Can you work these out from the model? Positions are in its coordinate system, mm. Round coordinates to 2 decimals unless told otherwise and drop trailing zeros. Order: outer loops, then holes, each group sorted by start corner. A loop starts at its lowest first (then second) coordinate and runs counter-clockwise, first axis right, second up. Notation, with made-up numbers: M -15,53 L 14,53 A11 ccw 14,74 Z; hole C 82.25,24.5 d3. An arc over 180 degrees is marked long. Answer as CSV lines item,"result". Start each with the question number.
from build123d import *

# Parameters (mm, degrees)
SKETCH1_W                   = 19.05
SKETCH1_H                   = 19.05
SKETCH1_W_2                 = 15.875
SKETCH1_H_2                 = 15.875
BOSS_EXTRUDE1_DEPTH         = 152.4
SKETCH2_R                   = 2.8956
BASEPLATE_MOUNT_HOLE_DEPTH  = 20.05
PS_BRACKET_MOUNT_HOLE_REACH = 21.05
SKETCH3_R                   = 4.7625
CUT_EXTRUDE1_REACH          = 21.05
SKETCH4_R                   = 4.7625
CUT_EXTRUDE2_REACH          = 21.05
SKETCH5_R                   = 4.7625


with BuildPart() as part:
    # Sketch1 → Boss-Extrude1 (new body, symmetric)
    with BuildSketch(Plane(origin=(0, 0, 0), x_dir=(0, -1, 0), z_dir=(0, 0, 1))):
        Rectangle(SKETCH1_W, SKETCH1_H)
        Rectangle(SKETCH1_W_2, SKETCH1_H_2, mode=Mode.SUBTRACT)
    extrude(amount=BOSS_EXTRUDE1_DEPTH, both=True)

    # Sketch2 → Baseplate Mount Hole (cut, through all)
    with BuildSketch(Plane(origin=(0, 9.525, 0), x_dir=(1, 0, 0), z_dir=(0, 1, 0))):
        with Locations((0, -114.3)):
            Circle(SKETCH2_R)
    extrude(amount=-BASEPLATE_MOUNT_HOLE_DEPTH, mode=Mode.SUBTRACT)

    # Sketch3 → PS Bracket Mount Hole (cut, up to next)
    with BuildSketch(Plane.ZY.offset(9.525), mode=Mode.PRIVATE) as ps_bracket_mount_hole_sk1:
        with Locations((-44.45, 0)):
            Circle(SKETCH3_R)
    ps_bracket_mount_hole_tool1 = extrude(ps_bracket_mount_hole_sk1.sketch, amount=-PS_BRACKET_MOUNT_HOLE_REACH, mode=Mode.PRIVATE) & part.part
    add(ps_bracket_mount_hole_tool1.solids().sort_by_distance((-9.525, 0, -44.45))[0], mode=Mode.SUBTRACT)

    # Sketch4 → Cut-Extrude1 (cut, up to next)
    with BuildSketch(Plane(origin=(0, 9.525, 0), x_dir=(1, 0, 0), z_dir=(0, 1, 0)), mode=Mode.PRIVATE) as cut_extrude1_sk1:
        with Locations((0, 21.200533333)):
            Circle(SKETCH4_R)
    cut_extrude1_tool1 = extrude(cut_extrude1_sk1.sketch, amount=-CUT_EXTRUDE1_REACH, mode=Mode.PRIVATE) & part.part
    add(cut_extrude1_tool1.solids().sort_by_distance((0, 9.525, -21.200533))[0], mode=Mode.SUBTRACT)

    # Sketch5 → Cut-Extrude2 (cut, up to next)
    with BuildSketch(Plane(origin=(9.525, 0, 0), x_dir=(0, 0, -1), z_dir=(1, 0, 0)), mode=Mode.PRIVATE) as cut_extrude2_sk1:
        with Locations((-89.0016, 0)):
            Circle(SKETCH5_R)
    cut_extrude2_tool1 = extrude(cut_extrude2_sk1.sketch, amount=-CUT_EXTRUDE2_REACH, mode=Mode.PRIVATE) & part.part
    add(cut_extrude2_tool1.solids().sort_by_distance((9.525, 0, 89.0016))[0], mode=Mode.SUBTRACT)


solid = part.part
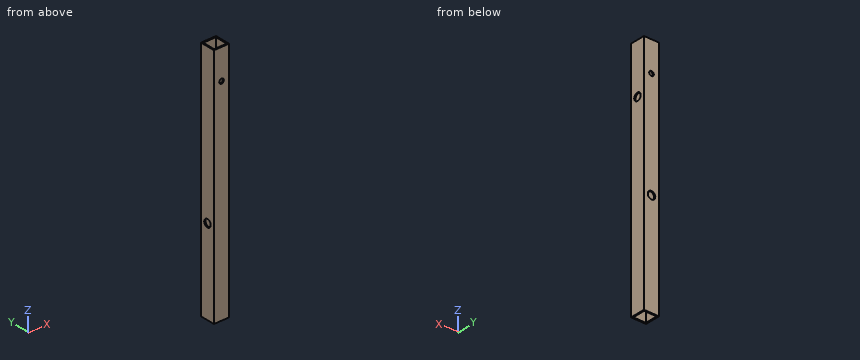
(1) I want a section at C-C on z = 114.3. Write out the boundary of the cut face in (x, y) (1 decimal), and give its area (3 significant figures).
(2) I want a section at D-D on z = -44.45. Write out the boundary of the cut face in (x, y) (1 decimal), and give its area (3 significant figures).
(3) I'm going to push flat-ended pins straight in: P1, Ø5.5, axis at x = 0, z = -21.2, coming from the +Y side; P2, Ø5, axis at x = 0, z = 114.3, coming from the -Y side. Where does each tip first touch, or does it pass through?
(4) I want a section at B-B on y = 0. Write out the boundary of the cut face in (x, z) (1 decimal).
(5) I want a section at A-A on x = 0. Write out the boundary of the cut face in (y, z) (1 decimal).
(6) If I drill on line 1 along Z through (x, y) = (0, 8.6); line 2 along Y through (x, z) = (3.25, 60) (1 decimal), over which ranges is the centre line in solid material (lowest first)?
From the geometry:
1,outline,"M -9.5,-9.5 L -2.9,-9.5 L -2.9,-7.9 L -7.9,-7.9 L -7.9,7.9 L -2.9,7.9 L -2.9,9.5 L -9.5,9.5 Z; M 2.9,-9.5 L 9.5,-9.5 L 9.5,9.5 L 2.9,9.5 L 2.9,7.9 L 7.9,7.9 L 7.9,-7.9 L 2.9,-7.9 Z"
1,area,"92.5 mm²"
2,outline,"M -9.5,-9.5 L 9.5,-9.5 L 9.5,9.5 L -9.5,9.5 L -9.5,4.8 L -7.9,4.8 L -7.9,7.9 L 7.9,7.9 L 7.9,-7.9 L -7.9,-7.9 L -7.9,-4.8 L -9.5,-4.8 Z"
2,area,"95.8 mm²"
3,P1,"y = -7.94"
3,P2,"through"
4,outline,"M -9.5,-152.4 L -7.9,-152.4 L -7.9,-49.2 L -9.5,-49.2 Z; M -9.5,-39.7 L -7.9,-39.7 L -7.9,152.4 L -9.5,152.4 Z; M 7.9,-152.4 L 9.5,-152.4 L 9.5,84.2 L 7.9,84.2 Z; M 7.9,93.8 L 9.5,93.8 L 9.5,152.4 L 7.9,152.4 Z"
5,outline,"M -9.5,-152.4 L -7.9,-152.4 L -7.9,111.4 L -9.5,111.4 Z; M -9.5,117.2 L -7.9,117.2 L -7.9,152.4 L -9.5,152.4 Z; M 7.9,-152.4 L 9.5,-152.4 L 9.5,-26 L 7.9,-26 Z; M 7.9,-16.4 L 9.5,-16.4 L 9.5,111.4 L 7.9,111.4 Z; M 7.9,117.2 L 9.5,117.2 L 9.5,152.4 L 7.9,152.4 Z"
6,line 1,"-152.4 to -25.96, -16.44 to 111.4, 117.2 to 152.4"
6,line 2,"-9.5 to -7.9, 7.9 to 9.5"
